The listing builds one solid part. Answer for the finished solid, in the listing's coordinates (mm). Face numbers are marked on the shaded views. A direction names the side the tool comes from. Give positions to 0.01 mm unless a question says otherwise; leave off trailing zeros. Write each loop counter-clockwise with the first axis right and the second up, starting at its lowest first coordinate (ties: lowest second). Pieces come first, ordered by that corner, then holes. Notation, with made-up numbers: (-7.5, 13) - (10.5, 13) arc R14 cw to (10.5, 37) - close; hole circle Ø6 at (5.25, 8.25). An arc over 180 degrees is marked (long way). Use a Markdown table: item, result. Add a question column.
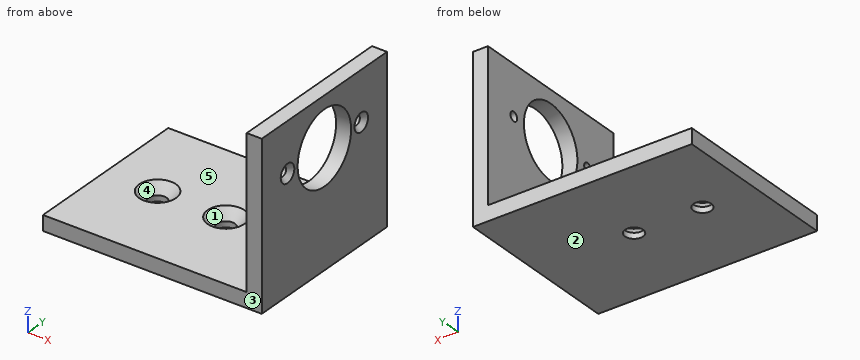
from build123d import *

# Parameters (mm, degrees)
F1_DEPTH       = 62
F3_D           = 26.5
F5_D           = 3.3
F5_CSINK_D     = 6.72
F5_CSINK_ANGLE = 90
F7_D           = 6.6
F7_CSINK_D     = 13.44
F7_CSINK_ANGLE = 90


with BuildPart() as f1:
    # F0 (on Front) → F1 (new body)
    with BuildSketch(Plane.XZ):
        Polygon((0, 5.5), (0, 0), (80, 0), (80, 60), (74.5, 60), (74.5, 5.5), align=None)
    extrude(amount=-F1_DEPTH)

    # F3 (through all)
    with Locations(Plane.YZ.offset(80)):
        with Locations((31, 42)):
            Hole(F3_D / 2)

    # F5 (through all)
    with Locations(Plane.YZ.offset(80)):
        with Locations((12.75, 42), (49.25, 42)):
            CounterSinkHole(F5_D / 2, F5_CSINK_D / 2, counter_sink_angle=F5_CSINK_ANGLE)

    # F7 (through all)
    with Locations(Plane.XY.offset(5.5)):
        with Locations((19, 31), (44, 31)):
            CounterSinkHole(F7_D / 2, F7_CSINK_D / 2, counter_sink_angle=F7_CSINK_ANGLE)


solid = f1.part
1. Consider L1, parallel to X at y = 31, z = 1.4; L2, parallel to Y at x = 19, z = 1.1; L3, parallel to Z at x = 76, y = 49. Determine where each line is inside the solid, lowest interval first. Write a range as [from, to].
2. The part is cut by section C-C (y = 31). Give the vertices of the cut face in (x, z).
3. For a pull along Y with two mould halves and no side action, classify the marked faces 1, 2 and 3 as released by +Y, released by -Y, zero draft, split by the parting line, or undercut.
4. The part is cut by section B-B (z = 42). Give the vertices of the cut face in (x, y).
5. The part is cut by section D-D (x = 19). Give the vertices of the cut face in (y, z), and give its area (3 significant figures).
6. The part is cut by section A-A (y = 12.75). Give the vertices of the cut face in (x, z), and give its area (3 significant figures).
7. Given P1, Ø5, axis at x = 52.5, y = 13, coming from the +Z side; P2, Ø24, axis at y = 31, z = 42, coming from the -X side; P3, Ø4, axis at y = 12.75, z = 42, coming from the +X side; P4, Ø3, axis at y = 55.5, z = 42.5, coming from the -X side, each flat-ended and moving along its own axis, determine where each tip first touches the part or whether it passes through.
8. Which of the six approach directions +Z, -Z, +X, -X, +Y, -Y give full straight-line access (tool end or side, diameter ignored) to the marked faces 4 and 5?
Check values:
| question | item | result |
|---|---|---|
| 1 | L1 | x = [0, 15.7], [22.3, 40.7], [47.3, 80] |
| 1 | L2 | y = [0, 27.7], [34.3, 62] |
| 1 | L3 | z = [0, 40.37], [43.63, 60] |
| 2 | outline | (0, 0) - (15.7, 0) - (15.7, 2.08) - (12.28, 5.5) - (0, 5.5) - close; (22.3, 0) - (40.7, 0) - (40.7, 2.08) - (37.28, 5.5) - (25.72, 5.5) - (22.3, 2.08) - close; (47.3, 0) - (80, 0) - (80, 28.75) - (74.5, 28.75) - (74.5, 5.5) - (50.72, 5.5) - (47.3, 2.08) - close; (74.5, 55.25) - (80, 55.25) - (80, 60) - (74.5, 60) - close |
| 3 | face 1 | undercut |
| 3 | face 2 | zero draft |
| 3 | face 3 | released by -Y |
| 4 | outline | (74.5, 0) - (80, 0) - (80, 9.39) - (78.29, 11.1) - (74.5, 11.1) - close; (74.5, 14.4) - (78.29, 14.4) - (80, 16.11) - (80, 17.75) - (74.5, 17.75) - close; (74.5, 44.25) - (80, 44.25) - (80, 45.89) - (78.29, 47.6) - (74.5, 47.6) - close; (74.5, 50.9) - (78.29, 50.9) - (80, 52.61) - (80, 62) - (74.5, 62) - close |
| 5 | outline | (0, 0) - (27.7, 0) - (27.7, 2.08) - (24.28, 5.5) - (0, 5.5) - close; (34.3, 0) - (62, 0) - (62, 5.5) - (37.72, 5.5) - (34.3, 2.08) - close |
| 5 | area | 293 mm2 |
| 6 | outline | (0, 0) - (80, 0) - (80, 38.64) - (78.29, 40.35) - (74.5, 40.35) - (74.5, 5.5) - (0, 5.5) - close; (74.5, 43.65) - (78.29, 43.65) - (80, 45.36) - (80, 60) - (74.5, 60) - close |
| 6 | area | 719 mm2 |
| 7 | P1 | stops at z = 5.5 |
| 7 | P2 | passes through |
| 7 | P3 | stops at x = 78.64 |
| 7 | P4 | stops at x = 74.5 |
| 8 | face 4 | +Z |
| 8 | face 5 | +Z, -X, +Y, -Y |
